Geometry check sheet. Reference: the model listing, model coordinates, mm. Face numbers are marked on the shaded views. A direction names the side the tool comes from. Round coordinates to 2 decimals unless told otherwise and drop trailing zeros. Loops run counter-clockwise (first coordinate to the right, second up) from the corner with the lowest first, then second, coordinate; pieces in that order, holes last.
```python
from build123d import *

# Parameters (mm, degrees)
BOSS_EXTRUDE1_DEPTH = 101.6
BOSS_EXTRUDE2_DEPTH = 0.3
CHAMFER1_SIZE       = 0.8


with BuildPart() as part:
    # Sketch1 → Boss-Extrude1 (new body)
    with BuildSketch(Plane.XY):
        with BuildLine():
            Line((-4.5, 0), (-4.5, -6.5))
            Line((-4.5, -6.5), (-6.5, -6.5))
            Line((-6.5, -6.5), (-6.5, 0))
            ThreePointArc((-6.5, 0), (0, 6.5), (6.5, 0))
            Line((6.5, 0), (6.5, -6.5))
            Line((6.5, -6.5), (4.5, -6.5))
            Line((4.5, -6.5), (4.5, 0))
            ThreePointArc((4.5, 0), (0, 4.5), (-4.5, 0))
        make_face()
    extrude(amount=BOSS_EXTRUDE1_DEPTH)

    # Sketch2 → Boss-Extrude2 (add)
    with BuildSketch(Plane(origin=(0, 0, 0), x_dir=(-1, 0, 0), z_dir=(0, 0, -1))):
        Polygon((4.5, 0), (4.5, -6.5), (-4.5, -6.5), (-4.5, 0), (-12.5, 0), (-12.5, -14.5), (12.5, -14.5), (12.5, 0), align=None)
    extrude(amount=-BOSS_EXTRUDE2_DEPTH)

    # Chamfer1
    chamfer1_edges = [part.edges().sort_by_distance(p)[0] for p in [
        (5.5, -6.5, 101.6),
        (6.5, -3.25, 101.6),
        (0, 6.5, 101.6),
        (-6.5, -3.25, 101.6),
        (-5.5, -6.5, 101.6),
        (-4.5, -3.25, 101.6),
        (0, 4.5, 101.6),
        (4.5, -3.25, 101.6),
    ]]
    chamfer(chamfer1_edges, length=CHAMFER1_SIZE)


solid = part.part
```
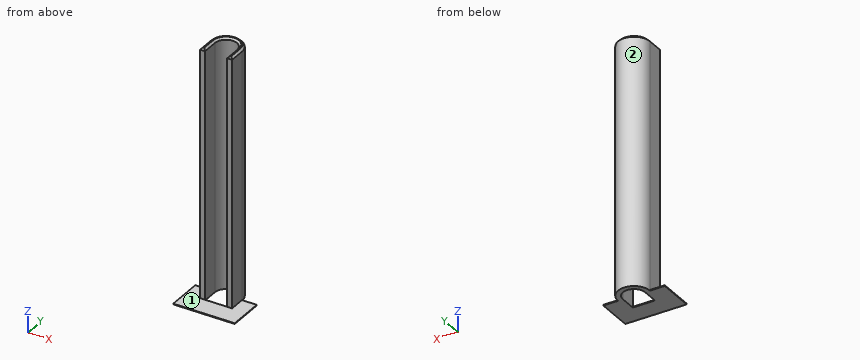
1) Sectioned sample at A-A, the plane x = 0. Record the cut outline in (y, z).
Report:
outline: (-14.5, 0) - (-6.5, 0) - (-6.5, 0.3) - (-14.5, 0.3) - close; (4.5, 0) - (6.5, 0) - (6.5, 100.8) - (5.7, 101.6) - (5.3, 101.6) - (4.5, 100.8) - close
2) Sectioned sample at B-B, the plane z = 92.5. Record the cut outline in (x, y).
Report:
outline: (-6.5, -6.5) - (-4.5, -6.5) - (-4.5, 0) arc R4.5 cw to (4.5, 0) - (4.5, -6.5) - (6.5, -6.5) - (6.5, 0) arc R6.5 ccw to (-6.5, 0) - close
3) Sectioned sample at C-C, the plane y = -10. Record the cut outline in (x, z).
Report:
outline: (-12.5, 0) - (12.5, 0) - (12.5, 0.3) - (-12.5, 0.3) - close
4) Scan lines: line 1 along X through (y, z) = (-2, 58.5); line 2 along Z through (x, y) = (-6.25, -12.25); line 3 along Y through (x, z) = (0, 54). Record each from-to range of solid material in increasing order.
Report:
line 1: x = -6.5 to -4.5, 4.5 to 6.5
line 2: z = 0 to 0.3
line 3: y = 4.5 to 6.5
5) Access from +Z, -Z, +X, -X, +Y, -Y to the whole of each face (thin tool, end or side, straight path). Record for the marked faces 1 and 2.
Report:
face 1: +Z, -Y
face 2: +Z, -Z, +Y
6) Gauge pin test, flat ends, axial feed: pin 1 (7 mm diameter, centred on y = -3, z = 50, fed in from +X); pin 2 (3 mm diameter, centred on y = -1.5, z = 37.5, fed in from -X); pin 3 (1 mm diameter, centred on x = 5.5, z = 88, fed in from +Y). Record the tip position at first contact, or that the pin passes through.
Report:
pin 1: stops at x = 6.5
pin 2: stops at x = -6.5
pin 3: stops at y = 4.15
